Part model, mm, in its own coordinate system. A direction names the side the tool comes from. Give positions to 0.01 mm unless a question says otherwise; leave off trailing zeros. Order: outer loops, then holes, each group sorted by start corner. A loop starts at its lowest first (then second) coordinate and runs counter-clockwise, first axis right, second up. Notation, with made-up numbers: (0, 79.5) - (35, 79.5) arc R13 cw to (35, 103.5) - close; hole circle Ø8 at (-8, -10.75). An arc over 180 degrees is marked (long way). Use a Markdown table: item, result. Add a question column.
from build123d import *

# Parameters (mm, degrees)
SKETCH1_R           = 15
BOSS_EXTRUDE1_DEPTH = 2
SKETCH2_R           = 7.5
SKETCH2_R_2         = 6.3
BOSS_EXTRUDE2_DEPTH = 14
SKETCH4_R           = 5
BOSS_EXTRUDE3_DEPTH = 42
SKETCH5_R           = 15
BOSS_EXTRUDE4_DEPTH = 3
SKETCH6_R           = 1.6
CUT_EXTRUDE1_DEPTH  = 3


with BuildPart() as part:
    # Sketch1 → Boss-Extrude1 (new body, symmetric)
    with BuildSketch(Plane(origin=(0, 0, 0), x_dir=(1, 0, 0), z_dir=(0, 1, 0))):
        Circle(SKETCH1_R)
    extrude(amount=BOSS_EXTRUDE1_DEPTH, both=True)

    # Sketch2 → Boss-Extrude2 (add)
    with BuildSketch(Plane.XZ.offset(2)):
        Circle(SKETCH2_R)
        Circle(SKETCH2_R_2, mode=Mode.SUBTRACT)
    extrude(amount=BOSS_EXTRUDE2_DEPTH)

    # Sketch4 → Boss-Extrude3 (add)
    with BuildSketch(Plane(origin=(0, 2, 0), x_dir=(1, 0, 0), z_dir=(0, 1, 0))):
        Circle(SKETCH4_R)
    extrude(amount=BOSS_EXTRUDE3_DEPTH)

    # Sketch5 → Boss-Extrude4 (add)
    with BuildSketch(Plane(origin=(0, 44, 0), x_dir=(1, 0, 0), z_dir=(0, 1, 0))):
        Circle(SKETCH5_R)
    extrude(amount=BOSS_EXTRUDE4_DEPTH)

    # Sketch6 → Cut-Extrude1 (cut)
    with BuildSketch(Plane(origin=(0, 47, 0), x_dir=(1, 0, 0), z_dir=(0, 1, 0))):
        with Locations((0, -11)):
            Circle(SKETCH6_R)
    extrude(amount=-CUT_EXTRUDE1_DEPTH, mode=Mode.SUBTRACT)


solid = part.part
1. Tool access for faces 5 (the face through (-14.985, 0.028, -0.66)), 6 (the face through (0, 47, 0)), 7 (the face through (-4, 2, -4)), 8 (the face through (0, -2, 0)), 9 (the face through (-0.35, 45.52, 12.56)): list every direction of +Z, -Z, +X, -X, +Y, -Y with a clear straight run to the whole face (end or side of a thin tool).
2. Cut at B-B (z = -9). Write the cut outline in (x, y), plus the area to 3 significant figures.
3. Cut at A-A (x = 0). Write the cut outline in (y, z).
4. Mould opens along Y. For faces 1 (the face through (-7.493, -8.902, 0.33)), 2 (the face through (-4, -2, -7)), 3 (the face through (-4, 44, -4)), 4 (the face through (-1.08, 22.71, 4.88)) say: released by +Y, released by -Y, zero draft, split by the parting line, or undercut.
5. Cut at C-C (z = 11). Write the cut outline in (x, y), plus the area to 3 significant figures.
6. Pin check, flat tips, straight feed: P1, Ø4, axis at y = 38.5, z = -5.5, coming from the +X side; P2, Ø3, axis at x = 4, y = 10, coming from the +Z side; P3, Ø5, axis at x = -11, z = 2, coming from the -Y side. Stop position of each tip, or through.
7. Cut at D-D (y = -6). Write the cut outline in (x, z).
8. Drill centre lines: probe 1 along Y at (x, z) = (9.25, 4.25); probe 2 along Z at (x, y) = (0, -6.25); probe 3 along Y at (x, z) = (2.5, 6.75). Where is each one in solid material? Low to high. Write a range as [from, to].
Responses:
| question | item | result |
|---|---|---|
| 1 | face 5 | +Y, -Y |
| 1 | face 6 | +Z, -Z, +X, -X, +Y |
| 1 | face 7 | none |
| 1 | face 8 | -Y |
| 1 | face 9 | +Y |
| 2 | outline | (-12, -2) - (12, -2) - (12, 2) - (-12, 2) - close; (-12, 44) - (12, 44) - (12, 47) - (-12, 47) - close |
| 2 | area | 168 mm² |
| 3 | outline | (-16, -7.5) - (-2, -7.5) - (-2, -15) - (2, -15) - (2, -5) - (44, -5) - (44, -15) - (47, -15) - (47, 9.4) - (44, 9.4) - (44, 5) - (2, 5) - (2, 15) - (-2, 15) - (-2, 7.5) - (-16, 7.5) - (-16, 6.3) - (-2, 6.3) - (-2, -6.3) - (-16, -6.3) - close; (44, 12.6) - (47, 12.6) - (47, 15) - (44, 15) - close |
| 4 | face 1 | zero draft |
| 4 | face 2 | released by -Y |
| 4 | face 3 | undercut |
| 4 | face 4 | undercut |
| 5 | outline | (-10.2, -2) - (10.2, -2) - (10.2, 2) - (-10.2, 2) - close; (-10.2, 44) - (-1.6, 44) - (-1.6, 47) - (-10.2, 47) - close; (1.6, 44) - (10.2, 44) - (10.2, 47) - (1.6, 47) - close |
| 5 | area | 133 mm² |
| 6 | P1 | stops at x = 3.57 |
| 6 | P2 | stops at z = 4.33 |
| 6 | P3 | stops at y = -2 |
| 7 | outline | circle Ø15 at (0, 0); hole circle Ø12.6 at (0, 0) |
| 8 | probe 1 | y = [-2, 2], [44, 47] |
| 8 | probe 2 | z = [-7.5, -6.3], [6.3, 7.5] |
| 8 | probe 3 | y = [-16, 2], [44, 47] |
